Geometry check sheet. Reference: the model listing, model coordinates, mm. A direction names the side the tool comes from. Give positions to 0.01 mm unless a question says otherwise; leave off trailing zeros. Order: outer loops, then holes, each group sorted by start corner. A loop starts at its lowest first (then second) coordinate and runs counter-clockwise, first axis right, second up. Notation, with made-up numbers: M 38,63 L 64,63 A19 ccw 64,77 Z; hole C 65,-22.75 d5. An arc over 180 degrees is marked long. Use CSV: the item, a comma, the result in double quotes. Start each with the question number.
from build123d import *

# Parameters (mm, degrees)
F1_DEPTH  = 25
F2_R      = 8
F3_R      = 10.95
F3_R_2    = 2.45
F5_DEPTH  = 1.25
F6_DEPTH  = 3
F4_R      = 12.7
F4_R_2    = 6.35
F8_DEPTH  = 1.25
F7_R      = 6.35
F9_DEPTH  = 1
F10_DEPTH = 3
F11_R     = 5
F7_R_2    = 2.5
F12_DEPTH = 3
F7_R_3    = 4.5
F13_DEPTH = 1
F14_R     = 0.99999
F15_R     = 12.5
F15_R_2   = 2.45
F16_DEPTH = 1
F17_R     = 0.99999


# Not quite as in the source:
# - a fillet or chamfer is up to 0.001 mm smaller than in the source, because OpenCascade refuses the exact size


with BuildPart() as f1:
    # F0 (on Front) → F1 (new body, symmetric)
    with BuildSketch(Plane.XZ):
        with BuildLine():
            Line((30, -25), (30, 25))
            Line((30, 25), (-30, 25))
            Line((-30, 25), (-30, 22))
            Line((-30, 22), (18, 22))
            ThreePointArc((18, 22), (24.3639610307, 19.3639610307), (27, 13))
            Line((27, 13), (27, -25))
            Line((27, -25), (30, -25))
        make_face()
    extrude(amount=F1_DEPTH, both=True)

    # F2
    f2_edges = [f1.edges().sort_by_distance(p)[0] for p in [
        (-30, -25, 23.5),
        (-30, 25, 23.5),
        (28.5, 25, -25),
        (28.5, -25, -25),
    ]]
    fillet(f2_edges, radius=F2_R)

    # F3 (on face) → F5 (cut)
    with BuildSketch(Plane.XY.offset(25)):
        with Locations((-3.6, 0)):
            Circle(F3_R)
        with Locations((-3.6, 0)):
            Circle(F3_R_2, mode=Mode.SUBTRACT)
    extrude(amount=-F5_DEPTH, mode=Mode.SUBTRACT)

    # F6 (cut): a face of the model
    f6_faces = [f1.faces().sort_by_distance(p)[0] for p in [
        (-3.6, 0, 25),
    ]]
    extrude(f6_faces, amount=-F6_DEPTH, mode=Mode.SUBTRACT)

    # F4 (on face) → F8 (cut)
    with BuildSketch(Plane.YZ.offset(30)):
        Circle(F4_R)
        Circle(F4_R_2, mode=Mode.SUBTRACT)
    extrude(amount=-F8_DEPTH, mode=Mode.SUBTRACT)

    # F7 (on face) → F9 (cut)
    with BuildSketch(Plane(origin=(27, 0, 0), x_dir=(0, -1, 0), z_dir=(-1, 0, 0))):
        with BuildLine():
            ThreePointArc((0, -12.7), (8.9802561211, -8.9802561211), (12.7, 0))
            ThreePointArc((12.7, 0), (-8.9802561211, 8.9802561211), (0, -12.7))
        make_face()
        Circle(F7_R, mode=Mode.SUBTRACT)
    extrude(amount=-F9_DEPTH, mode=Mode.SUBTRACT)

    # F10 (cut): a face of the model
    f10_faces = [f1.faces().sort_by_distance(p)[0] for p in [
        (30, 0, 0),
    ]]
    extrude(f10_faces, amount=-F10_DEPTH, mode=Mode.SUBTRACT)

    # F11
    f11_edges = [f1.edges().sort_by_distance(p)[0] for p in [
        (30, 0, 25),
    ]]
    fillet(f11_edges, radius=F11_R)

    # F7 (on face) → F12 (cut)
    with BuildSketch(Plane(origin=(27, 0, 0), x_dir=(0, -1, 0), z_dir=(-1, 0, 0))):
        with Locations((15.8969778568, -18.85)):
            Circle(F7_R_2)
    extrude(amount=-F12_DEPTH, mode=Mode.SUBTRACT)

    # F7 (on face) → F13 (join)
    with BuildSketch(Plane(origin=(27, 0, 0), x_dir=(0, -1, 0), z_dir=(-1, 0, 0))):
        with Locations((15.8969778568, -18.85)):
            Circle(F7_R_3)
        with Locations((15.8969778568, -18.85)):
            Circle(F7_R_2, mode=Mode.SUBTRACT)
    extrude(amount=F13_DEPTH)

    # F14 (radius 1 in the source; OpenCascade refuses exactly that, so slightly less here)
    f14_edges = [f1.edges().sort_by_distance(p)[0] for p in [
        (26, -11.396978, -18.85),
    ]]
    fillet(f14_edges, radius=F14_R)

    # F15 (on face) → F16 (join)
    with BuildSketch(Plane(origin=(0, 0, 22), x_dir=(1, 0, 0), z_dir=(0, 0, -1))):
        with Locations((-3.6, 0)):
            Circle(F15_R)
        with Locations((-3.6, 0)):
            Circle(F15_R_2, mode=Mode.SUBTRACT)
    extrude(amount=F16_DEPTH)

    # F17 (radius 1 in the source; OpenCascade refuses exactly that, so slightly less here)
    f17_edges = [f1.edges().sort_by_distance(p)[0] for p in [
        (-16.1, 0, 21),
    ]]
    fillet(f17_edges, radius=F17_R)


solid = f1.part
(1) Go/stop test with flat-tipped pins: P1, Ø12.5, axis at y = 0, z = 2.5, coming from the +X side; P2, Ø11.5, axis at y = 2.5, z = -3, coming from the -X side; P3, Ø14.5, axis at x = -14.5, y = -0.5, coming from the -Z side. Record where each tip stops, or that it passes through.
(2) Sectioned sample at B-B on z = -1. Record the cut outline in (x, y).
(3) Access from +Z, -Z, +X, -X, +Y, -Y to the whole of each face (thin tool, end or side, straight path). Record for faces 5 (the face through (30, 0, -13)), 6 (the face through (28, 6, -3)), 7 (the face through (28, 0, -25)), 8 (the face through (1.453, -9.715, 24.384)), 9 (the face through (-17, 0, 22)).
(4) Draft check along Z on faces 1 (the face through (26, -15, -16)), 2 (the face through (28.75, 3, 6)), 3 (the face through (-2, -11, 25)), 4 (the face through (27, 0, -14)). Enter one of: +Z half, -Z half, draft (parallel to the pull), parting line (faces both ways), or undercut.
(5) Sectioned sample at C-C on y = 19.5. Record the cut outline in (x, z), then the cut area to 3 significant figures.
(6) Thickness scan on line 1 (Y direction, x = -3.6, z = 24.4); line 2 (Y direction, x = 28.25, z = 0); line 3 (X direction, y = -12.5, z = 12). Record the ranges inside material, lowest first.
(7) Sectioned sample at D-D on z = -10.5. Record the cut outline in (x, y), then the cut area to 3 significant figures.
Responses:
1,P1,"x = 28.75"
1,P2,"x = 28"
1,P3,"z = 21"
2,outline,"M 27,-25 L 30,-25 L 30,-12.66 L 28.75,-12.66 L 28.75,-6.27 L 28,-6.27 L 28,-12.66 L 27,-12.66 Z; M 27,12.66 L 28,12.66 L 28,6.27 L 28.75,6.27 L 28.75,12.66 L 30,12.66 L 30,25 L 27,25 Z"
3,face 5,"+Z, -Z, +X, +Y, -Y"
3,face 6,"-X"
3,face 7,"-Z, +X, -X, +Y, -Y"
3,face 8,"+Z"
3,face 9,"-Z"
4,face 1,"draft"
4,face 2,"undercut"
4,face 3,"+Z half"
4,face 4,"undercut"
5,outline,"M -29.6,22 L 18,22 A9 cw 27,13 L 27,-24.6 L 30,-24.6 L 30,20 A5 ccw 25,25 L -29.6,25 Z"
5,area,"331 mm2"
6,line 1,"-25 to -10.95, 10.95 to 25"
6,line 2,"-25 to -6.35, 6.35 to 25"
6,line 3,"27 to 30"
7,outline,"M 27,-25 L 30,-25 L 30,-7.14 L 28.75,-7.14 L 28.75,7.14 L 30,7.14 L 30,25 L 27,25 L 27,7.14 L 28,7.14 L 28,-7.14 L 27,-7.14 Z"
7,area,"118 mm2"
